Answer from the drawing. Dimensions are ordinates in mm from the lowest x, y and z of the part. Give positions to 0.01 mm unless a question says otherwise; leave off trailing zeros. Write each loop counter-clockwise with the first axis right and the second up, starting at its lowest first coordinate (ties: lowest second). Pieces come first, ordered by that corner, then holes. Notation, with made-up numbers: (37, 72) -> (89, 72) arc R24 ccw to (89, 83) -> close; hole circle Ø10 at (-36.75, 7). An arc over 180 degrees is marked (long way). Write item = value, one per line.
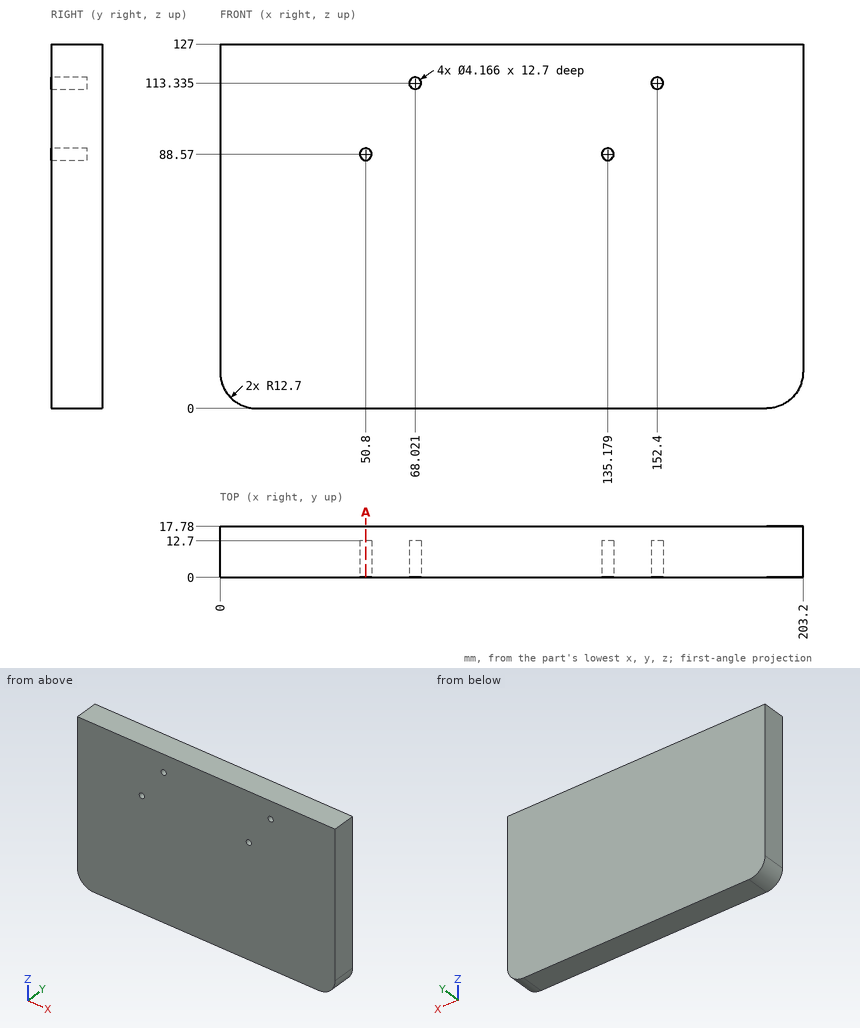
(1) Given P1, Ø2, axis at x = 174.5, z = 93, coming from the -Y side; P2, Ø2.5, axis at x = 152.4, z = 113.33, coming from the -Y side, each flat-ended and moving along its own axis, determine where each tip first touches the part or whether it passes through.
Checks:
P1 = 0
P2 = 12.7
(2) The part is cut by section A-A on x = 50.8. Determine the outline of the cut face in (y, z), plus the area to 4 significant figures.
Checks:
outline = (0, 0) -> (17.78, 0) -> (17.78, 127) -> (0, 127) -> (0, 90.65) -> (12.7, 90.65) -> (12.7, 86.49) -> (0, 86.49) -> close
area = 2,205 mm²
(3) Consider L1, parallel to X at y = 6.75, z = 111.5 (1 decimal). Determine where the line is inside the solid, lowest interval first.
Checks:
L1 = 0 to 67, 69 to 151.4, 153.4 to 203.2
